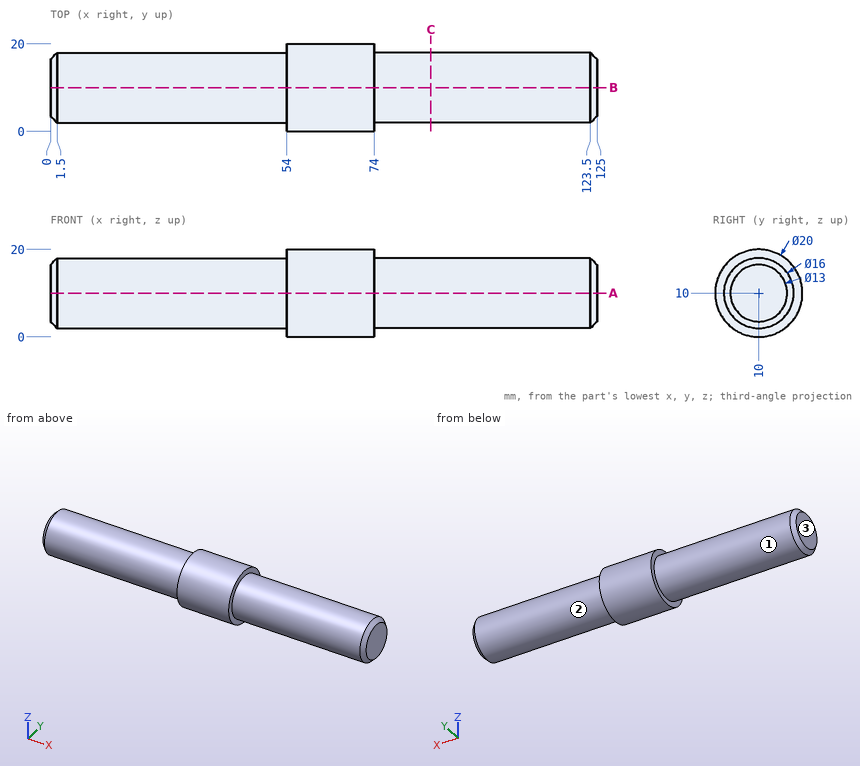
Job drawing, mm, ordinate dimensions from the low corner. One solid piece. A direction names the side the tool comes from. Round coordinates to 2 decimals unless told otherwise and drop trailing zeros. Loops run counter-clockwise (first coordinate to the right, second up) from the corner with the lowest first, then second, coordinate; pieces in that order, holes last. Notation, with made-up numbers: M 88.25,83.5 L 138.25,83.5 A17 ccw 138.25,115.5 Z; hole C -33.75,-21.75 d6. An arc over 180 degrees is marked long. One line per question, with ' | ' between items. Start each with the question number.
Item 1: Pin check, flat tips, straight feed: pin 1 Ø10 at (x, y) = (95.5, 11.5) entering from +Z; pin 2 Ø1 at (x, z) = (93, 6.5) entering from +Y; pin 3 Ø1.5 at (x, z) = (87.5, 4.5) entering from -Y. Stop position of each tip, or through.
Item 2: Which spindle directions (+Z, -Z, +X, -X, +Y, -Y) get a long thin tool onto all of the face, cutting with end or side? Do the marked faces 1, 2 and 3. Say none if no direction does.
Item 3: Cut at C-C, the plane x = 87. Write the cut outline in (y, z).
Item 4: Cut at A-A, the plane z = 10. Write the cut outline in (x, y), plus the area to 3 significant figures.
Item 5: Wall check: line 1 (X direction, y = 2.25, z = 7); line 2 (Y direction, x = 85.5, z = 10); line 3 (Y direction, x = 86, z = 4.25). Give the ranges that are in metal, low to high.
Responses:
1) pin 1: stops at z = 18 | pin 2: stops at y = 17.42 | pin 3: stops at y = 3.56
2) face 1: -X | face 2: +X | face 3: +Z, -Z, -X, +Y, -Y
3) outline: C 10,10 d16
4) outline: M 0,3.5 L 1.5,2 L 54,2 L 54,0 L 74,0 L 74,2 L 123.5,2 L 125,3.5 L 125,16.5 L 123.5,18 L 74,18 L 74,20 L 54,20 L 54,18 L 1.5,18 L 0,16.5 Z | area: 2,080 mm²
5) line 1: x = 54 to 74 | line 2: y = 2 to 18 | line 3: y = 4.44 to 15.56
